Work out the finished part from the listing and answer in its coordinate system (mm). A direction names the side the tool comes from. Round coordinates to 2 decimals unless told otherwise and drop trailing zeros. Loops run counter-clockwise (first coordinate to the right, second up) from the corner with the lowest first, then second, coordinate; pieces in that order, holes last.
```python
from build123d import *

# Parameters (mm, degrees)
SKETCH1_R             = 2
BOSS_EXTRUDE1_DEPTH   = 6.35
BOSS_EXTRUDE1_2_DEPTH = 6.35
SKETCH1_3_W           = 26.67
SKETCH1_3_H           = 12.446
BOSS_EXTRUDE2_DEPTH   = 61.976
SKETCH2_W             = 26.67
SKETCH2_H             = 12.446
SKETCH2_W_2           = 21.59
SKETCH2_H_2           = 7.366
BOSS_EXTRUDE3_DEPTH   = 13.97
SKETCH3_W             = 7.366
SKETCH3_H             = 6.985
CUT_EXTRUDE1_DEPTH    = 13.97


with BuildPart() as part:
    # Sketch1 → Boss-Extrude1 (new body)
    with BuildSketch(Plane(origin=(0, 0, 0), x_dir=(1, 0, 0), z_dir=(0, 1, 0))):
        with BuildLine():
            ThreePointArc((-13.335, 46.101), (-12.591051224, 47.897051224), (-10.795, 48.641))
            Line((-10.795, 48.641), (10.795, 48.641))
            ThreePointArc((10.795, 48.641), (12.591051224, 47.897051224), (13.335, 46.101))
            Line((13.335, 46.101), (13.335, 6.223))
            Line((13.335, 6.223), (-13.335, 6.223))
            Line((-13.335, 6.223), (-13.335, 46.101))
        make_face()
        with Locations(Location((0, 44.101004, 0), (0, 0, 270))):
            Circle(SKETCH1_R, mode=Mode.SUBTRACT)
    extrude(amount=BOSS_EXTRUDE1_DEPTH)



with BuildPart() as body_2:
    # Sketch1 → Boss-Extrude1 2 (new body)
    with BuildSketch(Plane(origin=(0, 0, 0), x_dir=(1, 0, 0), z_dir=(0, 1, 0))):
        with BuildLine():
            Line((-13.335, -6.223), (-13.335, -46.101))
            ThreePointArc((-13.335, -46.101), (-12.591051224, -47.897051224), (-10.795, -48.641))
            Line((-10.795, -48.641), (10.795, -48.641))
            ThreePointArc((10.795, -48.641), (12.591051224, -47.897051224), (13.335, -46.101))
            Line((13.335, -46.101), (13.335, -6.223))
            Line((13.335, -6.223), (-13.335, -6.223))
        make_face()
        with Locations(Location((0, -44.101004, 0), (0, 0, 270))):
            Circle(SKETCH1_R, mode=Mode.SUBTRACT)
    extrude(amount=BOSS_EXTRUDE1_2_DEPTH)


with BuildPart() as part_1:
    add(part.part)

    add(body_2.part)  # Boss-Extrude2 merges body 2
    # Sketch1_3 → Boss-Extrude2 (add)
    with BuildSketch(Plane(origin=(0, 0, 0), x_dir=(1, 0, 0), z_dir=(0, 1, 0))):
        Rectangle(SKETCH1_3_W, SKETCH1_3_H)
    extrude(amount=BOSS_EXTRUDE2_DEPTH)

    # Sketch2 → Boss-Extrude3 (add)
    with BuildSketch(Plane(origin=(0, 61.976, 0), x_dir=(1, 0, 0), z_dir=(0, 1, 0))):
        Rectangle(SKETCH2_W, SKETCH2_H)
        Rectangle(SKETCH2_W_2, SKETCH2_H_2, mode=Mode.SUBTRACT)
    extrude(amount=BOSS_EXTRUDE3_DEPTH)

    # Sketch3 → Cut-Extrude1 (cut)
    with BuildSketch(Plane(origin=(13.335, 0, 0), x_dir=(0, 0, -1), z_dir=(1, 0, 0))):
        with Locations((0, 65.4685)):
            Rectangle(SKETCH3_W, SKETCH3_H)
    extrude(amount=-CUT_EXTRUDE1_DEPTH, mode=Mode.SUBTRACT)


solid = part_1.part
```
1. Consider probe 1 along Z at (x, y) = (-0.5, 43.5); probe 2 along Y at (x, z) = (11.25, -21.5); probe 3 along Y at (x, z) = (2.5, -3). Determine where each line is inside the solid, lowest interval first.
Answer key:
probe 1: z = -6.22 to 6.22
probe 2: y = 0 to 6.35
probe 3: y = 0 to 61.98
2. Given pin 1 (3 mm diameter, centred on x = 0, z = -44.1, fed in from +Y); pin 2 (8 mm diameter, centred on x = -2, z = -29.5, fed in from +Y); pin 3 (4 mm diameter, centred on x = 4, y = 71.5, fed in from +Z); pin 4 (10 mm diameter, centred on x = -1, y = 38, fed in from -Z), each flat-ended and moving along its own axis, determine where each tip first touches the part or whether it passes through.
Answer key:
pin 1: passes through
pin 2: stops at y = 6.35
pin 3: stops at z = 6.22
pin 4: stops at z = -6.22
3. Determine the mould class of faces 4 (the face through (10.795, 72, 0)), 5 (the face through (12.57, 3.13, 47.92)), 6 (the face through (0, 0, -1)) for opening direction X: +X half, -X half, draft (parallel to the pull), parting line (faces both ways), or undercut.
Answer key:
face 4: undercut
face 5: +X half
face 6: draft
4. Which of the six approach directions +Z, -Z, +X, -X, +Y, -Y give full straight-line access (tool end or side, diameter ignored) to faces 1 (the face through (-10.795, 69, 0)), 2 (the face through (0, 6.35, 27)), 3 (the face through (0, 6.35, -28))?
Answer key:
face 1: +Y
face 2: +Z, +X, -X, +Y
face 3: -Z, +X, -X, +Y
5. Find section B-B (x = -8.25). Write down the section's boundary in (y, z).
Answer key:
outline: (0, -48.64) - (6.35, -48.64) - (6.35, -6.22) - (75.95, -6.22) - (75.95, -3.68) - (61.98, -3.68) - (61.98, 3.68) - (75.95, 3.68) - (75.95, 6.22) - (6.35, 6.22) - (6.35, 48.64) - (0, 48.64) - close
6. Find section C-C (y = 66). Write down the section's boundary in (x, z) (3 decimals), then the cut area to 3 significant figures.
Answer key:
outline: (-13.335, -6.223) - (13.335, -6.223) - (13.335, -3.683) - (-10.795, -3.683) - (-10.795, 3.683) - (13.335, 3.683) - (13.335, 6.223) - (-13.335, 6.223) - close
area: 154 mm2
7. Find section A-A (x = 0). Write down the section's boundary in (y, z).
Answer key:
outline: (0, -48.64) - (6.35, -48.64) - (6.35, -46.1) - (0, -46.1) - close; (0, -42.1) - (6.35, -42.1) - (6.35, -6.22) - (75.95, -6.22) - (75.95, -3.68) - (61.98, -3.68) - (61.98, 3.68) - (75.95, 3.68) - (75.95, 6.22) - (6.35, 6.22) - (6.35, 42.1) - (0, 42.1) - close; (0, 46.1) - (6.35, 46.1) - (6.35, 48.64) - (0, 48.64) - close
8. Find section D-D (z = 40). Write down the section's boundary in (x, y) (3 decimals).
Answer key:
outline: (-13.335, 0) - (13.335, 0) - (13.335, 6.35) - (-13.335, 6.35) - close
